Part model, mm, in its own coordinate system. A direction names the side the tool comes from. Round coordinates to 2 decimals unless told otherwise and drop trailing zeros. Loops run counter-clockwise (first coordinate to the right, second up) from the corner with the lowest first, then second, coordinate; pieces in that order, holes last. Notation, with made-up numbers: M -35,7.5 L 14,7.5 A19 ccw 14,25.5 Z; hole C -36.5,25 d7. An arc over 180 degrees is marked long. Answer as CSV lines item,"result". Start each with the question number.
Item 1: Which spindle directions (+Z, -Z, +X, -X, +Y, -Y) get a long thin tool onto all of the face, cutting with end or side? Do faces 4 (the flat face through (13, 51, -84.49)), 5 (the cylindrical face through (12.675, -2.649, -87.066)), 6 (the flat face through (-2, -16, 87)), 7 (the flat face through (-13, -17, 84.49)). Say none if no direction does.
Item 2: Mould opens along X. For faces 1 (the flat face through (-14, -35, -87)), 2 (the flat face through (25, -2, 0)), 3 (the cylindrical face through (-11.8, -27.1, 86.5)) say: pulls with the +X half, pulls with the -X half, needs draft (parallel to the pull), parting line crosses it, or undercut.
Item 3: Band-saw the part on B-B (y = 9). Give the cut face in (x, z), and give its area (3 significant figures).
Item 4: Wall check: line 1 (Z direction, x = 6, y = 89.5); line 2 (Y direction, x = -15.5, z = 14). Give the ranges that are in metal, low to high.
Item 5: Band-saw the part on C-C (x = -14). Give the cut face in (y, z).
Item 6: Drop flat-ended pins along their axis: pin 1 Ø1 at (x, z) = (-9, 10.5) entering from +Y; pin 2 Ø2 at (x, y) = (-1.5, -3) entering from +Z; pin 3 Ø2 at (y, z) = (48.5, -84.5) entering from -X. Give the stop position or say it passes through.
Item 7: Band-saw the part on A-A (y = 90). Give the cut face in (x, z), and give its area (3 significant figures).
Item 8: Band-saw the part on D-D (x = 5). Give the cut face in (y, z), and give its area (3 significant figures).
```python
from build123d import *

# Parameters (mm, degrees)
SKETCH_1_W                        = 50
SKETCH_1_H                        = 176.98019802
SM_BASE_FLANGE_1_DEPTH            = 4
SM_EDGE_FLANGE_1_STRIP_W          = 17.4732
SM_EDGE_FLANGE_1_STRIP_H          = 4
SM_EDGE_FLANGE_1_STRIP_CUT_DEPTH  = 25
SM_EDGE_FLANGE_1_RELIEF_W         = 19.4732
SM_EDGE_FLANGE_1_RELIEF_H         = 2
SM_EDGE_FLANGE_1_RELIEF_CUT_DEPTH = 4
SM_EDGE_FLANGE_1_DEPTH            = 25
SM_EDGE_FLANGE_2_STRIP_W          = 17.4732
SM_EDGE_FLANGE_2_STRIP_H          = 4
SM_EDGE_FLANGE_2_STRIP_CUT_DEPTH  = 25
SM_EDGE_FLANGE_2_RELIEF_W         = 19.4732
SM_EDGE_FLANGE_2_RELIEF_H         = 2
SM_EDGE_FLANGE_2_RELIEF_CUT_DEPTH = 4
SM_EDGE_FLANGE_2_DEPTH            = 25
SM_EDGE_FLANGE_3_STRIP_W          = 17.4732
SM_EDGE_FLANGE_3_STRIP_H          = 4
SM_EDGE_FLANGE_3_STRIP_CUT_DEPTH  = 23
SM_EDGE_FLANGE_3_DEPTH            = 23
SM_EDGE_FLANGE_4_STRIP_W          = 17.4732
SM_EDGE_FLANGE_4_STRIP_H          = 4
SM_EDGE_FLANGE_4_STRIP_CUT_DEPTH  = 23
SM_EDGE_FLANGE_4_DEPTH            = 23
SKETCH_18_R                       = 5
CUT_EXTRUDE_1_DEPTH               = 205.809644527
SKETCH_19_R                       = 5
CUT_EXTRUDE_2_DEPTH               = 205.809644527
CHAMFER_1_SIZE                    = 3
CHAMFER_2_SIZE                    = 3


# Sheet-metal steps are written as plain solids
with BuildPart() as part:
    # Sketch 1 → 基体-法兰1 (new body)
    with BuildSketch(Plane(origin=(0, 0, 0), x_dir=(1, 0, 0), z_dir=(0, 1, 0))):
        Rectangle(SKETCH_1_W, SKETCH_1_H)
    extrude(amount=-SM_BASE_FLANGE_1_DEPTH)

    # 边线-法兰1 strip (across the edge) → 边线-法兰1 strip cut (cut)
    with BuildSketch(Plane(origin=(25, 0, -88.49009901), x_dir=(0, 0, 1), z_dir=(-1, 0, 0))):
        with Locations((-4, -2)):
            Rectangle(SM_EDGE_FLANGE_1_STRIP_W, SM_EDGE_FLANGE_1_STRIP_H)
    extrude(amount=SM_EDGE_FLANGE_1_STRIP_CUT_DEPTH, mode=Mode.SUBTRACT)

    # 边线-法兰1 relief (on the sheet) → 边线-法兰1 relief cut (cut)
    with BuildSketch(Plane(origin=(25, 0, -83.75349901), x_dir=(0, 0, 1), z_dir=(0, 1, 0))):
        with Locations((-7.7366, -26)):
            Rectangle(SM_EDGE_FLANGE_1_RELIEF_W, SM_EDGE_FLANGE_1_RELIEF_H)
    extrude(amount=-SM_EDGE_FLANGE_1_RELIEF_CUT_DEPTH, mode=Mode.SUBTRACT)

    # 边线-法兰1 section (across the edge) → 边线-法兰1 (add)
    with BuildSketch(Plane(origin=(25, 0, -88.49009901), x_dir=(0, 0, 1), z_dir=(-1, 0, 0))):
        with BuildLine():
            Line((0, 0.7366), (0, 100))
            Line((0, 100), (4, 100))
            Line((4, 100), (4, 0.7366))
            ThreePointArc((4, 0.7366), (4.215745145, 0.215745145), (4.7366, 0))
            Line((4.7366, 0), (4.7366, -4))
            ThreePointArc((4.7366, -4), (1.38731802, -2.61268198), (0, 0.7366))
        make_face()
    extrude(amount=SM_EDGE_FLANGE_1_DEPTH)

    # 边线-法兰2 strip (across the edge) → 边线-法兰2 strip cut (cut)
    with BuildSketch(Plane(origin=(0, 0, 88.49009901), x_dir=(0, 0, -1), z_dir=(1, 0, 0))):
        with Locations((-4, -2)):
            Rectangle(SM_EDGE_FLANGE_2_STRIP_W, SM_EDGE_FLANGE_2_STRIP_H)
    extrude(amount=SM_EDGE_FLANGE_2_STRIP_CUT_DEPTH, mode=Mode.SUBTRACT)

    # 边线-法兰2 relief (on the sheet) → 边线-法兰2 relief cut (cut)
    with BuildSketch(Plane(origin=(0, 0, 83.75349901), x_dir=(0, 0, -1), z_dir=(0, 1, 0))):
        with Locations((-7.7366, 1)):
            Rectangle(SM_EDGE_FLANGE_2_RELIEF_W, SM_EDGE_FLANGE_2_RELIEF_H)
    extrude(amount=-SM_EDGE_FLANGE_2_RELIEF_CUT_DEPTH, mode=Mode.SUBTRACT)

    # 边线-法兰2 section (across the edge) → 边线-法兰2 (add)
    with BuildSketch(Plane(origin=(0, 0, 88.49009901), x_dir=(0, 0, -1), z_dir=(1, 0, 0))):
        with BuildLine():
            Line((0, 0.7366), (0, 100))
            Line((0, 100), (4, 100))
            Line((4, 100), (4, 0.7366))
            ThreePointArc((4, 0.7366), (4.215745145, 0.215745145), (4.7366, 0))
            Line((4.7366, 0), (4.7366, -4))
            ThreePointArc((4.7366, -4), (1.38731802, -2.61268198), (0, 0.7366))
        make_face()
    extrude(amount=SM_EDGE_FLANGE_2_DEPTH)

    # 边线-法兰3 strip (across the edge) → 边线-法兰3 strip cut (cut)
    with BuildSketch(Plane(origin=(-2, -4, 88.49009901), x_dir=(0, 0, -1), z_dir=(-1, 0, 0))):
        with Locations((-4, -2)):
            Rectangle(SM_EDGE_FLANGE_3_STRIP_W, SM_EDGE_FLANGE_3_STRIP_H)
    extrude(amount=SM_EDGE_FLANGE_3_STRIP_CUT_DEPTH, mode=Mode.SUBTRACT)

    # 边线-法兰3 section (across the edge) → 边线-法兰3 (add)
    with BuildSketch(Plane(origin=(-2, -4, 88.49009901), x_dir=(0, 0, -1), z_dir=(-1, 0, 0))):
        with BuildLine():
            Line((0, 0.7366), (0, 31))
            Line((0, 31), (4, 31))
            Line((4, 31), (4, 0.7366))
            ThreePointArc((4, 0.7366), (4.215745145, 0.215745145), (4.7366, 0))
            Line((4.7366, 0), (4.7366, -4))
            ThreePointArc((4.7366, -4), (1.38731802, -2.61268198), (0, 0.7366))
        make_face()
    extrude(amount=SM_EDGE_FLANGE_3_DEPTH)

    # 边线-法兰4 strip (across the edge) → 边线-法兰4 strip cut (cut)
    with BuildSketch(Plane(origin=(-25, -4, -88.49009901), x_dir=(0, 0, 1), z_dir=(1, 0, 0))):
        with Locations((-4, -2)):
            Rectangle(SM_EDGE_FLANGE_4_STRIP_W, SM_EDGE_FLANGE_4_STRIP_H)
    extrude(amount=SM_EDGE_FLANGE_4_STRIP_CUT_DEPTH, mode=Mode.SUBTRACT)

    # 边线-法兰4 section (across the edge) → 边线-法兰4 (add)
    with BuildSketch(Plane(origin=(-25, -4, -88.49009901), x_dir=(0, 0, 1), z_dir=(1, 0, 0))):
        with BuildLine():
            Line((0, 0.7366), (0, 31))
            Line((0, 31), (4, 31))
            Line((4, 31), (4, 0.7366))
            ThreePointArc((4, 0.7366), (4.215745145, 0.215745145), (4.7366, 0))
            Line((4.7366, 0), (4.7366, -4))
            ThreePointArc((4.7366, -4), (1.38731802, -2.61268198), (0, 0.7366))
        make_face()
    extrude(amount=SM_EDGE_FLANGE_4_DEPTH)

    # 草图18 → 切除-拉伸1 (cut, through all)
    with BuildSketch(Plane.XY.offset(88.49009901)):
        with Locations((-14.061160699, -22.641783907)):
            Circle(SKETCH_18_R)
    extrude(amount=-CUT_EXTRUDE_1_DEPTH, mode=Mode.SUBTRACT)

    # 草图19 → 切除-拉伸2 (cut, through all)
    with BuildSketch(Plane.XY.offset(88.49009901)):
        with Locations((12.330904878, 90)):
            Circle(SKETCH_19_R)
    extrude(amount=-CUT_EXTRUDE_2_DEPTH, mode=Mode.SUBTRACT)

    # 倒角1
    chamfer_1_edges = [part.edges().sort_by_distance(p)[0] for p in [
        (-2, -35, 86.49009901),
        (-25, -35, 86.49009901),
        (-25, -35, -86.49009901),
        (-2, -35, -86.49009901),
    ]]
    chamfer(chamfer_1_edges, length=CHAMFER_1_SIZE)

    # 倒角2
    chamfer_2_edges = [part.edges().sort_by_distance(p)[0] for p in [
        (25, 100, -86.49009901),
        (0, 100, -86.49009901),
        (0, 100, 86.49009901),
        (25, 100, 86.49009901),
    ]]
    chamfer(chamfer_2_edges, length=CHAMFER_2_SIZE)


solid = part.part
```
Answer block:
1,face 4,"+X, -X, +Y"
1,face 5,"-Z, +X, -Y"
1,face 6,"+Z, +Y, -Y"
1,face 7,"+X, -X, -Y"
2,face 1,"needs draft"
2,face 2,"pulls with the +X half"
2,face 3,"undercut"
3,outline,"M 0,-88.49 L 25,-88.49 L 25,-84.49 L 0,-84.49 Z; M 0,84.49 L 25,84.49 L 25,88.49 L 0,88.49 Z"
3,area,"200 mm^2"
4,line 1,"z = -88.49 to -84.49, 84.49 to 88.49"
4,line 2,"y = -4 to 0"
5,outline,"M -35,-88.49 L -27.64,-88.49 L -27.64,-84.49 L -35,-84.49 Z; M -35,84.49 L -27.64,84.49 L -27.64,88.49 L -35,88.49 Z; M -17.64,-88.49 L -4.74,-88.49 A4.74 ccw 0,-83.75 L 0,83.75 A4.74 ccw -4.74,88.49 L -17.64,88.49 L -17.64,84.49 L -4.74,84.49 A0.74 cw -4,83.75 L -4,-83.75 A0.74 cw -4.74,-84.49 L -17.64,-84.49 Z"
6,pin 1,"stops at y = 0"
6,pin 2,"stops at z = 88.41"
6,pin 3,"stops at x = 0"
7,outline,"M 0,-88.49 L 7.33,-88.49 L 7.33,-84.49 L 0,-84.49 Z; M 0,84.49 L 7.33,84.49 L 7.33,88.49 L 0,88.49 Z; M 17.33,-88.49 L 25,-88.49 L 25,-84.49 L 17.33,-84.49 Z; M 17.33,84.49 L 25,84.49 L 25,88.49 L 17.33,88.49 Z"
7,area,"120 mm^2"
8,outline,"M -4,-83.75 A4.74 ccw 0.74,-88.49 L 100,-88.49 L 100,-84.49 L 0.74,-84.49 A0.74 cw 0,-83.75 L 0,83.75 A0.74 cw 0.74,84.49 L 100,84.49 L 100,88.49 L 0.74,88.49 A4.74 ccw -4,83.75 Z"
8,area,"1,500 mm^2"
